Could you check a few things on this model? Use its own coordinates, in mm. Coordinates: 2 decimals unless noted, no trailing zeros. Loops run counter-clockwise (first coordinate to the right, second up) from the corner with the lowest first, then second, coordinate; pieces in that order, holes last. Notation, with made-up numbers: (-9.5, 72) -> (36.5, 72) arc R19 ccw to (36.5, 79) -> close; hole circle Ø3 at (44.25, 38). An arc over 180 degrees is marked (long way). One line per question, with ' | ' between items.
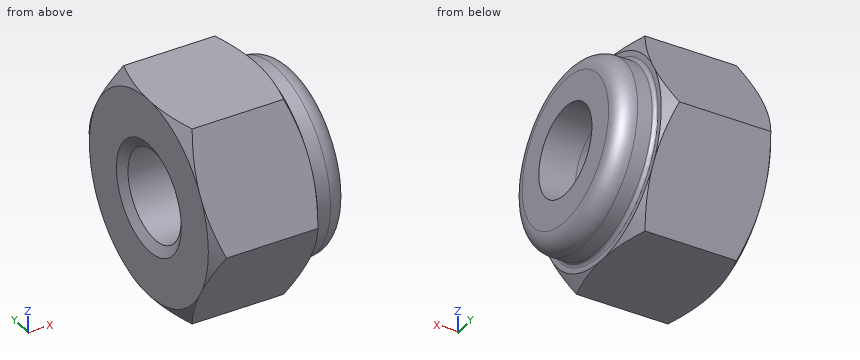
Autodesk Inventor part; units mm, degrees
ref_plane "Work Plane1" through (8.9209, 0, 0) normal (0, 0.8660254, -0.5) x (-1, 0, 0)
ref_plane "Work Plane2" through (1.5, 0, 0) normal (1, 0, 0) x (0, 0, -1)
ref_plane "YZ Plane" through (0, 0, 0) normal (1, 0, 0) x (0, 1, 0)
sketch "Sketch1" plane through (0, 0, 0) normal (1, 0, 0) x (0, 1, 0)
  line L0 (3.1754, 0) -> (1.5877, -2.75)
  line L1 (1.5877, -2.75) -> (-1.5877, -2.75)
  line L2 (-1.5877, -2.75) -> (-3.1754, 0)
  line L3 (-3.1754, 0) -> (-1.5877, 2.75)
  line L4 (-1.5877, 2.75) -> (1.5877, 2.75)
  line L5 (1.5877, 2.75) -> (3.1754, 0)
  point P0 (0, 0)
  point P1 (0, 0)
  dimension "d0" = 6.3509
extrude "Body" add sketch "Sketch1" along normal blind 3
sketch "Sketch2" plane through (0, 0, 0) normal (-1, 0, 0) x (0, 0, 1)
  point P0 (0, 0)
hole "Thread" at (0, 0, 0) direction (1, 0, 0) diameter 2.459 end through all
chamfer "Chamfer1" distance 0.2706 angle 30 1 edges at (0, 0, -1.2295) measured on face at (0, -1.925, -1.1495)
sketch "Sketch3" plane through (0, 0, 0) normal (0, 0, 1) x (1, 0, 0)
  line L0 (0, 3.1754) -> (3, 3.1754)
  line L1 (3, 1.5877) -> (3, 3.1754)
  line L2 (-0.48, 0) -> (2.88, 0)
  line L3 (2.7544, 3.1754) -> (3, 2.75)
  dimension "d3" = 5.5
  dimension "d4" = 30
revolve "Chamfer3" cut sketch "Sketch3" angle 360 about axis through (-10, 0, 0) along (1, 0, 0)
ref_plane "Work Plane1" through (8.9209, 0, 0) normal (0, 0.8660254, -0.5) x (-1, 0, 0)
ref_plane "Work Plane2" through (1.5, 0, 0) normal (1, 0, 0) x (0, 0, -1)
mirror "Mirror1" about plane through (1.5, 0, 0) normal (1, 0, 0) of "Chamfer3"
sketch "Sketch6" plane through (3, 0, 0) normal (1, 0, 0) x (0, 0, -1)
  circle A0 centre (0, 0) radius 1.2295
  circle A1 centre (0, 0) radius 2.5
  dimension "d26" = 5
extrude "Extrusion2" add sketch "Sketch6" along normal blind 1
fillet "Fillet1" radius 0.5 1 edges at (4, 0, 2.5)
fillet "Fillet2" radius 0.1 1 edges at (3, 0, 2.5)
equation "\"d0\" = 1.1547 * SW"
equation "\"d13\" = -0.5 * GD1 + 0.5 * NND"
equation "\"d21\" = -0.5 * GD1 + 0.5 * NND"
equation "\"d3\" = SW01"
equation "\"d4\" = ANG2"
equation "\"ANG2\" = 30deg"
equation "\"NND\" = 3"
equation "\"KOH\" = 2.4"
equation "\"SW\" = 5.5"
equation "\"SW01\" = SW"
equation "\"GUL\" = 0.541266 * PTC"
equation "\"TOA\" = 30deg"
equation "\"PTC\" = 0.5"
equation "\"E0\" = 1.155 * SW"
equation "\"THREADDIA\" = 3"
equation "\"GAL\" = 0.541266 * PTC"
properties part number "M3 Nylon Nut" material "Stainless Steel"
1) If we section it at A-A on x = 3.35: Please give me the cut outline in (y, z), and give its area (3 significant figures).
Data:
outline: circle Ø5 at (0, 0); hole circle Ø2.46 at (0, 0) | area: 14.9 mm²
2) I need wall thicknesses on line 1 along Z through (x, y) = (1.3, 0); line 2 along Z through (x, y) = (3.3, -2); line 3 along Y through (x, z) = (3.15, 1.1) (3 decimals). Which ranges of each line are inside material? Lowest first, please. Write a range as from..to.
Data:
line 1: -2.75..-1.23, 1.23..2.75 | line 2: -1.5..1.5 | line 3: -2.245..-0.549, 0.549..2.245
3) I'm going to push a flat-ended pin straight in: pin 1 Ø1 at (x, z) = (2, 1.5) entering from -Y. Where does the tip first touch, or does it pass through?
Data:
pin 1: y = -2.6
